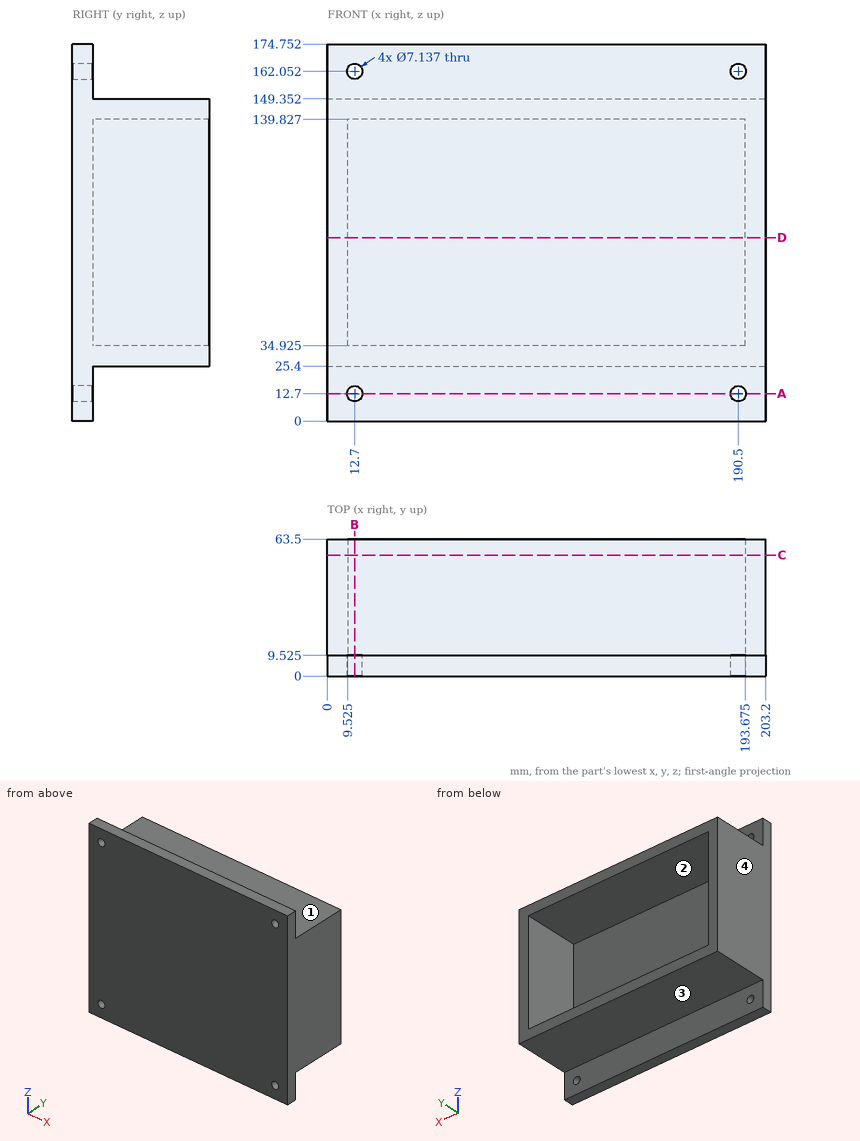
Check sheet for the drawn part. Datum: minimum x, y, z corner. Units: mm. A direction names the side the tool comes from. Coordinates: 2 decimals unless noted, no trailing zeros. Loops run counter-clockwise (first coordinate to the right, second up) from the corner with the lowest first, then second, coordinate; pieces in that order, holes last. Notation, with made-up numbers: (14, -1.75) -> (67, -1.75) arc R26 cw to (67, 35.25) -> close; hole circle Ø7 at (-23, -8.5). An arc over 180 degrees is marked (long way). Answer in a Markdown table with one row per item.
1. Material ranges on line 1 along X through (y, z) = (3, 12.7); line 2 along Z through (x, y) = (190.5, 2.5); line 3 along X through (y, z) = (51, 129) (1 decimal), recorded low to high. Write a range as [from, to].
Check values:
| item | result |
|---|---|
| line 1 | x = [0, 9.13], [16.27, 186.93], [194.07, 203.2] |
| line 2 | z = [0, 9.13], [16.27, 158.48], [165.62, 174.75] |
| line 3 | x = [0, 9.5], [193.7, 203.2] |
2. Sectioned sample at D-D, the plane z = 85. Record the boundary of the cut face in (x, y) (1 decimal).
Check values:
| item | result |
|---|---|
| outline | (0, 0) -> (203.2, 0) -> (203.2, 63.5) -> (193.7, 63.5) -> (193.7, 9.5) -> (9.5, 9.5) -> (9.5, 63.5) -> (0, 63.5) -> close |
3. Go/stop test with flat-tipped pins: pin 1 (8 mm diameter, centred on x = 190.5, z = 162.052, fed in from +Y) (3 decimals); pin 2 (20.5 mm diameter, centred on x = 84.5, z = 15.5, fed in from +Y); pin 3 (12 mm diameter, centred on x = 76, y = 46.5, fed in from +Z); pin 4 (4.5 mm diameter, centred on x = 12.7, z = 12.7, fed in from -Y). Record where each tip stops, or that it passes through.
Check values:
| item | result |
|---|---|
| pin 1 | stops at y = 9.525 |
| pin 2 | stops at y = 63.5 |
| pin 3 | stops at z = 149.35 |
| pin 4 | passes through |
4. Sectioned sample at A-A, the plane z = 12.7. Record the boundary of the cut face in (x, y) (1 decimal).
Check values:
| item | result |
|---|---|
| outline | (0, 0) -> (9.1, 0) -> (9.1, 9.5) -> (0, 9.5) -> close; (16.3, 0) -> (186.9, 0) -> (186.9, 9.5) -> (16.3, 9.5) -> close; (194.1, 0) -> (203.2, 0) -> (203.2, 9.5) -> (194.1, 9.5) -> close |
5. Sectioned sample at B-B, the plane x = 12.7. Record the boundary of the cut face in (y, z) (1 decimal).
Check values:
| item | result |
|---|---|
| outline | (0, 0) -> (9.5, 0) -> (9.5, 9.1) -> (0, 9.1) -> close; (0, 16.3) -> (9.5, 16.3) -> (9.5, 25.4) -> (63.5, 25.4) -> (63.5, 34.9) -> (9.5, 34.9) -> (9.5, 139.8) -> (63.5, 139.8) -> (63.5, 149.4) -> (9.5, 149.4) -> (9.5, 158.5) -> (0, 158.5) -> close; (0, 165.6) -> (9.5, 165.6) -> (9.5, 174.8) -> (0, 174.8) -> close |
6. Access from +Z, -Z, +X, -X, +Y, -Y to the whole of each face (thin tool, end or side, straight path). Record for the marked faces 1, 2, 3 and 4.
Check values:
| item | result |
|---|---|
| face 1 | +Z, +X, -X, +Y |
| face 2 | +Y |
| face 3 | -Z, +X, -X, +Y |
| face 4 | +Z, -Z, -X, +Y, -Y |
7. Sectioned sample at C-C, the plane y = 56. Record the boundary of the cut face in (x, z) (1 decimal), then the cut area to 3 significant figures.
Check values:
| item | result |
|---|---|
| outline | (0, 25.4) -> (203.2, 25.4) -> (203.2, 149.4) -> (0, 149.4) -> close; hole (9.5, 34.9) -> (193.7, 34.9) -> (193.7, 139.8) -> (9.5, 139.8) -> close |
| area | 5,870 mm2 |
